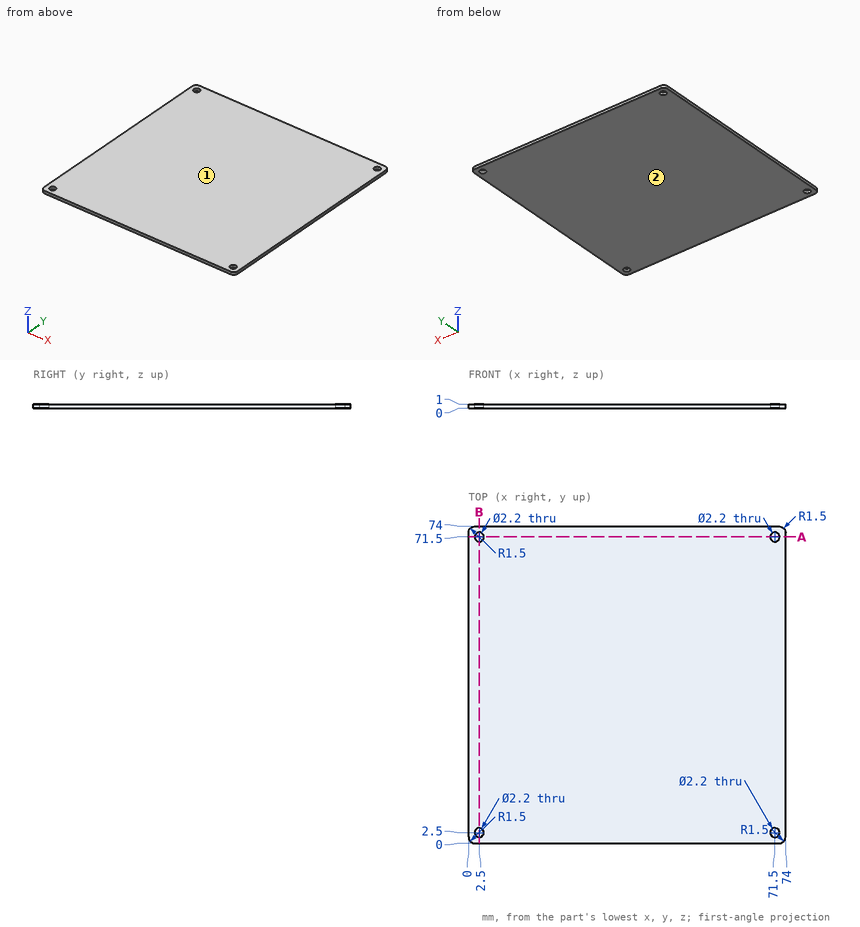
Here's the drawing with two shaded views (mm, measured from the low corner). I have some questions. Coordinates: 2 decimals unless noted, no trailing zeros. Write each loop counter-clockwise with the first axis right and the second up, starting at its lowest first coordinate (ties: lowest second). Pieces come first, ordered by that corner, then holes. Notation, with made-up numbers: (19.5, 74) -> (33.5, 74) arc R31 cw to (33.5, 100) -> close; hole circle Ø3 at (-5.75, 75). An arc over 180 degrees is marked (long way). Write item = value, one per line. Start each with the question number.
(1) I want a section at A-A (y = 71.5). Please give me the cut outline in (x, z).
(2) We'd pull the mould along Z, two halves only. Please class the marked faces 1 and 2: released by +Z, released by -Z, zero draft, split by the parting line, or undercut.
(3) I need wall thicknesses on line 1 (Y direction, x = 2.5, z = 0.6); line 2 (X direction, y = 71, z = 0.5). Which ranges of each line are inside material? Lowest first, please. Write a range as [from, to].
Result set:
q1.outline = (0, 0) -> (1.4, 0) -> (1.4, 1) -> (0, 1) -> close; (3.6, 0) -> (70.4, 0) -> (70.4, 1) -> (3.6, 1) -> close; (72.6, 0) -> (74, 0) -> (74, 1) -> (72.6, 1) -> close
q2.face_1 = released by +Z
q2.face_2 = released by -Z
q3.line_1 = [0, 1.4], [3.6, 70.4], [72.6, 74]
q3.line_2 = [0, 1.52], [3.48, 70.52], [72.48, 74]
